For this review, take the finished solid that the model builds, in its own axes (mm). Face numbers are marked on the shaded views. A direction names the side the tool comes from. Give positions to 0.01 mm unless a question says otherwise; leave off trailing zeros. Write each loop counter-clockwise with the first axis right and the second up, starting at its lowest first coordinate (ties: lowest second). Pieces come first, ordered by that corner, then holes. Notation, with made-up numbers: M -20.75,34.5 L -5.75,34.5 A28 ccw -5.75,73.5 Z; hole C 31.5,-35.5 d9. An arc over 180 degrees is marked long. One line per item, written item: value. Start each with the question number.
Item 1: Consider section B-B, the plane x = 0. Write out the cut boundary in (y, z).
Item 2: Clearance check with flat-ended pins moving along their axes: pin 1 Ø3 at (x, z) = (15, 10.5) entering from -Y; pin 2 Ø3 at (y, z) = (14, 4.5) entering from -X; pin 3 Ø4 at (x, z) = (9, 3) entering from -Y. State where each tip first meets the part, or that it passes through.
Item 3: Tool access review of the marked faces 1, 2, 3, 4 and 5: name each direction out of +Z, -Z, +X, -X, +Y, -Y from which nothing blocks a thin tool from reaching the whole face with its end or side.
Item 4: To check wall thickness, follow probe 1 along X at (y, z) = (-8, 4.75) (3 decimals); probe 2 along X at (y, z) = (7, 3.5); probe 3 along Y at (x, z) = (39, 13.25). State the ranges of each line that lie inside material, in increasing order.
Item 5: Mouldability with a two-part tool opening along Y and no side actions: class the marked faces 6, 7 and 8 as released by +Y, released by -Y, zero draft, split by the parting line, or undercut.
Item 6: Consider section D-D, the plane y = 8. Give the number of separate pieces and of enclosed holes in the cut face, and give its area (3 significant figures).
```python
from build123d import *

# Parameters (mm, degrees)
SKETCH_3_R          = 2.55
SKETCH_3_R_2        = 1.55
EXTRUDE_1_DEPTH     = 5
SKETCH_4_R          = 1.55
EXTRUDE_2_DEPTH     = 9.25
FILLET_2_R          = 2
FILLET_START        = 6.9999999
FILLET_3_2_DEPTH    = 8.0000001
SKETCH_5_W          = 7
SKETCH_5_H          = 6
CUT_EXTRUDE_1_DEPTH = 2.6
SKETCH_6_R          = 7.55
CUT_EXTRUDE_2_DEPTH = 62.147874109
EXTRUDE_START       = 2.6
SKETCH_7_W          = 7
SKETCH_7_H          = 0.15
EXTRUDE_3_DEPTH     = 2.6


with BuildPart() as part:
    # 草图3 → 凸台-拉伸1 (new body)
    with BuildSketch(Plane.XY):
        with BuildLine():
            Line((13, 20), (-5, 9.797958971))
            ThreePointArc((-5, 9.797958971), (-11, 0), (-5, -9.797958971))
            Line((-5, -9.797958971), (13, -20))
            Line((13, -20), (34, -20))
            ThreePointArc((34, -20), (41.071067812, -17.071067812), (44, -10))
            Line((44, -10), (44, 10))
            ThreePointArc((44, 10), (41.071067812, 17.071067812), (34, 20))
            Line((34, 20), (13, 20))
        make_face()
        Circle(SKETCH_3_R, mode=Mode.SUBTRACT)
        with Locations((16.975, -8)):
            Circle(SKETCH_3_R_2, mode=Mode.SUBTRACT)
        with Locations((16.975, 8)):
            Circle(SKETCH_3_R_2, mode=Mode.SUBTRACT)
        with Locations((40.025, 8)):
            Circle(SKETCH_3_R_2, mode=Mode.SUBTRACT)
        with Locations((40.025, -8)):
            Circle(SKETCH_3_R_2, mode=Mode.SUBTRACT)
    extrude(amount=EXTRUDE_1_DEPTH)

    # 草图4 → 凸台-拉伸2 (add)
    with BuildSketch(Plane.XY.offset(5)):
        with BuildLine():
            Line((13, -15), (13, 15))
            Line((13, 15), (13, 20))
            Line((13, 20), (18, 20))
            Line((18, 20), (34, 20))
            ThreePointArc((34, 20), (41.071067812, 17.071067812), (44, 10))
            Line((44, 10), (44, -10))
            ThreePointArc((44, -10), (41.071067812, -17.071067812), (34, -20))
            Line((34, -20), (18, -20))
            Line((18, -20), (13, -20))
            Line((13, -20), (13, -15))
        make_face()
        with Locations((16.975, 8)):
            Circle(SKETCH_4_R, mode=Mode.SUBTRACT)
        with Locations((16.975, -8)):
            Circle(SKETCH_4_R, mode=Mode.SUBTRACT)
        with Locations((40.025, -8)):
            Circle(SKETCH_4_R, mode=Mode.SUBTRACT)
        with Locations((40.025, 8)):
            Circle(SKETCH_4_R, mode=Mode.SUBTRACT)
    extrude(amount=EXTRUDE_2_DEPTH)

    # 圆角2
    fillet_2_edges = [part.edges().sort_by_distance(p)[0] for p in [
        (13, 0, 5),
    ]]
    fillet(fillet_2_edges, radius=FILLET_2_R)

    # 圆角3: read off the stored shape, not the designer's step
    # 圆角3 outline → 圆角3 (revolve, cut)
    with BuildSketch(Plane(origin=(11, 0, 7), x_dir=(1, 0, 0), z_dir=(0, 0, 1))):
        with BuildLine():
            ThreePointArc((7, -20), (3.464466094, -18.535533906), (2, -15))
            Line((2, -15), (2, -20))
            Line((2, -20), (7, -20))
        make_face()
        with BuildLine():
            Line((2, 20), (2, 15))
            ThreePointArc((2, 15), (3.464466094, 18.535533906), (7, 20))
            Line((7, 20), (2, 20))
        make_face()
    revolve(axis=Axis((11, 0, 7), (0, 1, 0)), mode=Mode.SUBTRACT)

    # Fillet 3 2 outline → Fillet 3 2 (cut)
    with BuildSketch(Plane.XY.offset(FILLET_START)):
        with BuildLine():
            Line((13, -20), (18, -20))
            ThreePointArc((18, -20), (14.464466094, -18.535533906), (13, -15))
            Line((13, -15), (13, -20))
        make_face()
        with BuildLine():
            Line((13, 20), (13, 15))
            ThreePointArc((13, 15), (14.464466094, 18.535533906), (18, 20))
            Line((18, 20), (13, 20))
        make_face()
    extrude(amount=FILLET_3_2_DEPTH, mode=Mode.SUBTRACT)

    # 草图5 → 切除-拉伸1 (cut)
    with BuildSketch(Plane(origin=(0, 0, 8.5), x_dir=(-1, 0, 0), z_dir=(0, 0, -1))):
        with Locations((-40.5, 8)):
            Rectangle(SKETCH_5_W, SKETCH_5_H)
        with Locations((-40.5, -8)):
            Rectangle(SKETCH_5_W, SKETCH_5_H)
        with Locations((-16.5, -8)):
            Rectangle(SKETCH_5_W, SKETCH_5_H)
        with Locations((-16.5, 8)):
            Rectangle(SKETCH_5_W, SKETCH_5_H)
    extrude(amount=-CUT_EXTRUDE_1_DEPTH, mode=Mode.SUBTRACT)

    # 草图6 → 切除-拉伸2 (cut, through all)
    with BuildSketch(Plane.XZ.offset(20)):
        with Locations((28.5, 14.5)):
            Circle(SKETCH_6_R)
    extrude(amount=-CUT_EXTRUDE_2_DEPTH, mode=Mode.SUBTRACT)

    # 草图7 → 凸台-拉伸3 (add)
    with BuildSketch(Plane(origin=(0, 0, 11.1), x_dir=(-1, 0, 0), z_dir=(0, 0, -1)).offset(EXTRUDE_START)):
        with BuildLine():
            Line((-37, 11), (-43.949874371, 11))
            ThreePointArc((-43.949874371, 11), (-43.957124407, 10.925026241), (-43.963809512, 10.85))
            Line((-43.963809512, 10.85), (-37, 10.85))
            Line((-37, 10.85), (-37, 11))
        make_face()
        with Locations((-40.5, 5.075)):
            Rectangle(SKETCH_7_W, SKETCH_7_H)
        with Locations((-40.5, -5.075)):
            Rectangle(SKETCH_7_W, SKETCH_7_H)
        with BuildLine():
            Line((-37, -11), (-37, -10.85))
            Line((-37, -10.85), (-43.963809512, -10.85))
            ThreePointArc((-43.963809512, -10.85), (-43.957124407, -10.925026241), (-43.949874371, -11))
            Line((-43.949874371, -11), (-37, -11))
        make_face()
        with Locations((-16.5, -10.925)):
            Rectangle(SKETCH_7_W, SKETCH_7_H)
        with Locations((-16.5, -5.075)):
            Rectangle(SKETCH_7_W, SKETCH_7_H)
        with Locations((-16.5, 5.075)):
            Rectangle(SKETCH_7_W, SKETCH_7_H)
        with Locations((-16.5, 10.925)):
            Rectangle(SKETCH_7_W, SKETCH_7_H)
    extrude(amount=-EXTRUDE_3_DEPTH)


solid = part.part
```
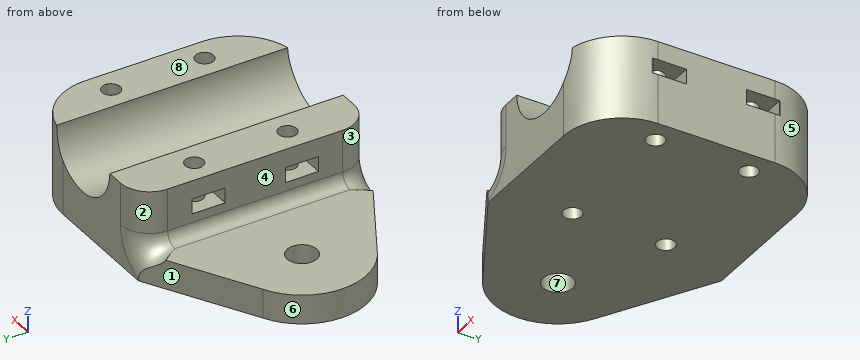
Model answer:
1. outline: M -12.63,0 L -2.55,0 L -2.55,5 L -12.63,5 Z; M 2.55,0 L 12.63,0 L 12.63,5 L 2.55,5 Z
2. pin 1: stops at y = -19.77
2. pin 2: stops at x = -0.23
2. pin 3: stops at y = -18.87
3. face 1: +Z, -Z, -X, +Y
3. face 2: +Z, -X, +Y
3. face 3: +Z, -X, -Y
3. face 4: +Z, -X, +Y, -Y
3. face 5: +Z, -Z, +X, +Y
4. probe 1: x = -7.55 to 15.425, 18.525 to 38.475, 41.575 to 44
4. probe 2: x = -8.49 to 15.79, 18.16 to 38.84, 41.21 to 44
4. probe 3: y = -18.66 to -9.16, -6.84 to 6.84, 9.16 to 18.66
5. face 6: split by the parting line
5. face 7: undercut
5. face 8: zero draft
6. separate pieces: 5
6. enclosed holes: 0
6. area: 351 mm2
